Can you work these out from the model? Positions are in its coordinate system, mm. A direction names the side the tool comes from. Coordinates: 2 decimals unless noted, no trailing zeros. Loops run counter-clockwise (first coordinate to the right, second up) from the corner with the lowest first, then second, coordinate; pieces in that order, holes last. Notation, with made-up numbers: (83.5, -33.5) -> (103.5, -33.5) arc R21 cw to (103.5, -6.5) -> close; hole circle Ø11 at (-10.5, 81.5). An arc over 180 degrees is marked (long way). Put each result on its own line as item: value. Start each with the question number.
Item 1: If we section it at B-B on y = 22: Please give me the cut outline in (x, z), plus the area to 3 significant figures.
Item 2: For faces 1 (the flat face through (4.762, 43, 417)), 2 (the flat face through (4.6, 24.2, 819.15)), which set-ups out of +Z, -Z, +X, -X, +Y, -Y let a thin tool reach every point of the face, with its end or its side?
Item 3: Will these pins go through, and if not, where does the flat tip stop? P1, Ø18, axis at x = 31, z = 512, coming from the +Y side; P2, Ø5, axis at y = 30, z = 244.5, coming from the +X side; P3, Ø2, axis at y = 10.5, z = 545.5, coming from the +X side.
Item 4: Please list where these lines run through material, in increasing order: L1, parallel to Y at x = 35.5, z = 471; L2, parallel to Y at x = 3.5, z = 167. Write a range as from..to.
Item 5: If we section it at A-A on z = 506: Please give me the cut outline in (x, y).
Autodesk Inventor part; units mm, degrees
ref_plane "Start plane" through (0, 0, 25.4) normal (0, 0, 1) x (1, 0, 0)
ref_plane "End plane" through (0, 0, 819.15) normal (0, 0, 1) x (1, 0, 0)
ref_plane "Work Plane3" through (400.05, 0, 819.15) normal (0, 0, 1) x (1, 0, 0)
ref_plane "Start plane" through (0, 0, 25.4) normal (0, 0, 1) x (1, 0, 0)
ref_plane "End plane" through (0, 0, 819.15) normal (0, 0, 1) x (1, 0, 0)
sketch "Sketch" plane through (0, 0, 0) normal (0, 0, 1) x (1, 0, 0)
  line L0 (0, 76.2) -> (0, 0)
  line L1 (0, 0) -> (50.8, 0)
  line L2 (50.8, 0) -> (50.8, 2.7625)
  line L3 (48.8, 4.7625) -> (12.6365, 4.7625)
  line L4 (4.7625, 12.6365) -> (4.7625, 74.2)
  line L5 (2.7625, 76.2) -> (0, 76.2)
  line L6 (-7.0414, 0) -> (21.5385, 0) construction
  line L7 (0, -8.0414) -> (0, 34.5385) construction
  arc A0 (4.7625, 12.6365) -> (12.6365, 4.7625) centre (12.6365, 12.6365) ccw
  arc A1 (50.8, 2.7625) -> (48.8, 4.7625) centre (48.8, 2.7625) ccw
  arc A2 (4.7625, 74.2) -> (2.7625, 76.2) centre (2.7625, 74.2) ccw
  line L8 (0, 93.5453) -> (0, -24.9725) construction
  line L9 (-18.6925, 0) -> (62.8653, 0) construction
  point P0 (50.8, 4.7625)
  point P1 (4.7625, 4.7625)
  point P2 (4.7625, 76.2)
  dimension "d12" = 4.7625
  dimension "d13" = 76.2
  dimension "d14" = 50.8
  dimension "d15" = 0
  dimension "d16" = 4.7625
  dimension "d17" = 0
  dimension "d18" = 7.874
  dimension "d19" = 2
extrude "Body" add sketch "Sketch" along normal up to surface (793.75 mm away) from surface at 25.4
sketch "Sketch3" plane through (0, 0, 0) normal (0, 0, 1) x (1, 0, 0)
  line L0 (0, 0) -> (10, 0)
ref_plane "Work Plane5" through (0, 0, 0) normal (0, -1, 0) x (1, 0, 0)
sketch "Sketch4" plane through (0, 0, 0) normal (0, -1, 0) x (1, 0, 0)
  line L0 (-2, 25.4) -> (12, 25.4)
  line L1 (-2, 819.15) -> (12, 819.15)
  dimension "d23" = 793.75
ref_plane "Work Plane3" through (400.05, 0, 819.15) normal (0, 0, 1) x (1, 0, 0)
split "Split1" plane through (400.05, 0, 819.15) removes the side toward (0, 0, 1)
ref_plane "Work Plane4" through (-923.925, 0, 25.4) normal (0, 0, -1) x (-1, 0, 0)
split "Split2" plane through (-923.925, 0, 25.4) removes the side toward (0, 0, -1)
equation "\"d12\" = G_T"
equation "\"d13\" = G_H"
equation "\"d14\" = G_W"
equation "\"d16\" = G_T"
equation "\"d18\" = G_IR"
equation "\"d4\" = G_L"
equation "\"G_W\" = 50.8"
equation "\"G_H\" = 76.2"
equation "\"G_T\" = 4.7625"
equation "\"G_ER\" = 4.064"
equation "\"G_IR\" = 7.874"
equation "\"G_L\" = d23"
equation "\"ex\" = 0"
equation "\"ey\" = 0"
equation "\"G_OFFSET_START\" = -25.4"
equation "\"G_OFFSET_END\" = -25.4"
equation "\"d20\" = -G_OFFSET_START"
equation "\"d21\" = G_OFFSET_END + B_L"
equation "\"B_L\" = 844.55"
properties part number "ANSI L 3 x 2 x 3_16 00000005"
Solutions:
1. outline: (0, 25.4) -> (4.76, 25.4) -> (4.76, 819.15) -> (0, 819.15) -> close
1. area: 3,780 mm^2
2. face 1: +Z, -Z, +X, +Y
2. face 2: +Z, +X, -X, +Y, -Y
3. P1: y = 4.76
3. P2: x = 4.76
3. P3: x = 5.41
4. L1: 0..4.76
4. L2: 0..76.06
5. outline: (0, 0) -> (50.8, 0) -> (50.8, 2.76) arc R2 ccw to (48.8, 4.76) -> (12.64, 4.76) arc R7.87 cw to (4.76, 12.64) -> (4.76, 74.2) arc R2 ccw to (2.76, 76.2) -> (0, 76.2) -> close
